CAD build for the part. Positions are in the model's coordinates, mm. Face numbers are marked on the shaded views. A direction names the side the tool comes from. Coordinates: 2 decimals unless noted, no trailing zeros. Write each loop counter-clockwise with the first axis right and the second up, starting at its lowest first coordinate (ties: lowest second). Pieces come first, ordered by that corner, then holes. Notation, with made-up numbers: (-18.5, 50) - (19.5, 50) arc R19 ccw to (19.5, 87) - close; hole circle Ø7 at (-1, 35). An arc over 180 degrees is marked (long way). One line per question, with ' | ' between items. Start each with the question number.
1. Probe line 1 (Y direction, x = -16, z = 24); line 2 (X direction, y = 45, z = 7); line 3 (Y direction, x = -2, z = 27). List the from-to ranges inside material, lowest first.
2. Two-plate mould, pull along Y, no slides. Class the marked faces 1, 2, 3 and 4: +Y half, -Y half, draft (parallel to the pull), parting line (faces both ways), or undercut.
3. Band-saw the part on B-B, the plane x = 13. Write the cut outline in (y, z).
4. Which spindle directions (+Z, -Z, +X, -X, +Y, -Y) get a long thin tool onto all of the face, cutting with end or side? Do the marked faces 5, 6, 7 and 8. Say none if no direction does.
5. Flat gauge pins, fed straight in: P1, Ø2.5, axis at x = -28, y = 35.5, coming from the +Z side; P2, Ø2.5, axis at x = -28, z = 19.5, coming from the -Y side; P3, Ø2.5, axis at x = -27.5, z = 16.5, coming from the +Y side. Where does each tip first touch, or does it go through?
6. Band-saw the part on C-C, the plane x = -19.5. Write the cut outline in (y, z), then the cut area to 3 significant figures.
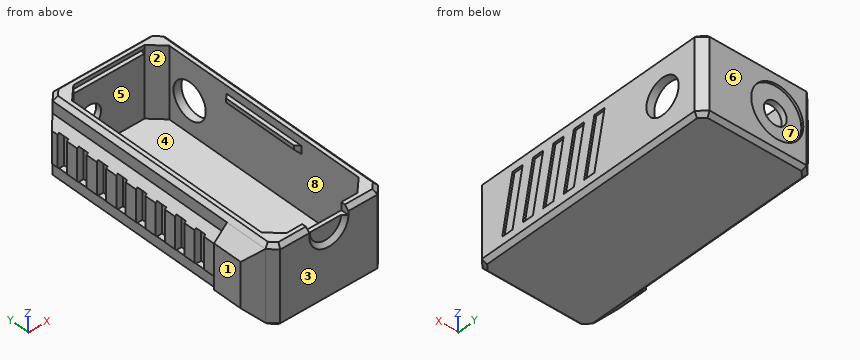
from build123d import *

# Parameters (mm, degrees)
F2_W      = 52
F2_H      = 116
F2_W_2    = 44.8
F2_H_2    = 108.8
F3_DEPTH  = 36
F4_DEPTH  = 3.6
F7_SIZE   = 3.6
F8_SIZE   = 5.9976
F6_R      = 5.25
F9_DEPTH  = 3.6
F5_R      = 8.25
F10_DEPTH = 3.6
F11_W     = 18
F11_H     = 3.6
F12_DEPTH = 3.6
F13_W     = 32.8048
F13_H     = 2
F14_DEPTH = 2.1
F6_R_2    = 12
F15_DEPTH = 1
F16_R     = 0.5
F17_W     = 38.28
F17_H     = 3.6
F19_DEPTH = 1.8
F18_W     = 38.28
F18_H     = 3.6
F20_DEPTH = 1.8
F21_SIZE  = 1.79999
F23_DEPTH = 1.8
F24_SIZE  = 1.79999
F26_W     = 89.2
F26_H     = 21.6
F27_DEPTH = 3.6
F28_DEPTH = 5.9976
F30_SIZE  = 3.59999
F29_W     = 4.775
F29_H     = 15.6718
F31_DEPTH = 2.9972
F32_SIZE  = 5.99759
F34_DEPTH = 0.9


# Not quite as in the source:
# - two fillets or chamfers of one size are made in one step
# - a fillet or chamfer is up to 0.001 mm smaller than in the source, because OpenCascade refuses the exact size


with BuildPart() as f3:
    # F2 (on Top) → F3 (new body)
    with BuildSketch(Plane.XY):
        Rectangle(F2_W, F2_H)
        Rectangle(F2_W_2, F2_H_2, mode=Mode.SUBTRACT)
    extrude(amount=F3_DEPTH)

    # F2 (on Top) → F4 (join)
    with BuildSketch(Plane.XY):
        Rectangle(F2_W_2, F2_H_2)
    extrude(amount=F4_DEPTH)

    # F7
    f7_edges = [f3.edges().sort_by_distance(p)[0] for p in [
        (-26, -58, 18),
        (26, -58, 18),
        (26, 58, 18),
        (-26, 58, 18),
    ]]
    chamfer(f7_edges, length=F7_SIZE)

    # F8
    f8_edges = [f3.edges().sort_by_distance(p)[0] for p in [
        (-22.4, 54.4, 19.8),
        (22.4, 54.4, 19.8),
        (-22.4, -54.4, 19.8),
        (22.4, -54.4, 19.8),
    ]]
    chamfer(f8_edges, length=F8_SIZE)

    # F6 (on face) → F9 (cut)
    with BuildSketch(Plane(origin=(0, 58, 0), x_dir=(-1, 0, 0), z_dir=(0, 1, 0))):
        with Locations((8.84, 18)):
            Circle(F6_R)
    extrude(amount=-F9_DEPTH, mode=Mode.SUBTRACT)

    # F5 (on face) → F10 (cut)
    with BuildSketch(Plane.YZ.offset(26)):
        with Locations((38, 18)):
            Circle(F5_R)
    extrude(amount=-F10_DEPTH, mode=Mode.SUBTRACT)

    # F11 (on face) → F12 (cut)
    with BuildSketch(Plane.XZ.offset(58)):
        with Locations((0, 34.2)):
            Rectangle(F11_W, F11_H)
    extrude(amount=-F12_DEPTH, mode=Mode.SUBTRACT)

    # F13 (on face) → F14 (cut)
    with BuildSketch(Plane.XZ.offset(-54.4)):
        with Locations((0, 33.2)):
            Rectangle(F13_W, F13_H)
    extrude(amount=-F14_DEPTH, mode=Mode.SUBTRACT)

    # F6 (on face) → F15 (cut)
    with BuildSketch(Plane(origin=(0, 58, 0), x_dir=(-1, 0, 0), z_dir=(0, 1, 0))):
        with Locations((8.84, 18)):
            Circle(F6_R_2)
        with Locations((8.84, 18)):
            Circle(F6_R, mode=Mode.SUBTRACT)
    extrude(amount=-F15_DEPTH, mode=Mode.SUBTRACT)

    # F16
    f16_edges = [f3.edges().sort_by_distance(p)[0] for p in [
        (0, 56.5, 34.2),
    ]]
    fillet(f16_edges, radius=F16_R)

    # F17 (on face) → F19 (join)
    with BuildSketch(Plane(origin=(22.4, 0, 0), x_dir=(0, -1, 0), z_dir=(-1, 0, 0))):
        with Locations((0, 30.6)):
            Rectangle(F17_W, F17_H)
    extrude(amount=F19_DEPTH)

    # F18 (on face) → F20 (join)
    with BuildSketch(Plane.YZ.offset(-22.4)):
        with Locations((0, 30.6)):
            Rectangle(F18_W, F18_H)
    extrude(amount=F20_DEPTH)

    # F21 (size 1.8 in the source; OpenCascade refuses exactly that, so slightly less here)
    f21_edges = [f3.edges().sort_by_distance(p)[0] for p in [
        (-20.6, -19.14, 30.6),
        (-20.6, 0, 28.8),
        (-20.6, 19.14, 30.6),
        (20.6, 19.14, 30.6),
        (20.6, 0, 28.8),
        (20.6, -19.14, 30.6),
        (-15.7, -58, 36),
        (-24.2, -56.2, 36),
        (-26, 0, 36),
        (-24.2, 56.2, 36),
        (0, 58, 36),
        (24.2, 56.2, 36),
        (26, 0, 36),
        (24.2, -56.2, 36),
        (15.7, -58, 36),
        (0, -58, 0),
        (-24.2, -56.2, 0),
        (-26, 0, 0),
        (-24.2, 56.2, 0),
        (0, 58, 0),
        (24.2, 56.2, 0),
        (26, 0, 0),
        (24.2, -56.2, 0),
    ]]
    chamfer(f21_edges, length=F21_SIZE)

    # F11 (on face) → F23 (cut)
    with BuildSketch(Plane.XZ.offset(58)):
        with BuildLine():
            ThreePointArc((-9, 32.4), (0, 23.4), (9, 32.4))
            Line((9, 32.4), (-9, 32.4))
        make_face()
    extrude(amount=-F23_DEPTH, mode=Mode.SUBTRACT)

    # F24 (size 1.8 in the source; OpenCascade refuses exactly that, so slightly less here)
    f24_edges = [f3.edges().sort_by_distance(p)[0] for p in [
        (0, -56.2, 23.4),
    ]]
    chamfer(f24_edges, length=F24_SIZE)

    # F26 (on face) → F27 (join)
    with BuildSketch(Plane(origin=(-26, 0, 0), x_dir=(0, -1, 0), z_dir=(-1, 0, 0))):
        with Locations((-9.8, 18)):
            Rectangle(F26_W, F26_H)
    extrude(amount=F27_DEPTH)

    # F26 (on face) → F28 (join)
    with BuildSketch(Plane(origin=(-26, 0, 0), x_dir=(0, -1, 0), z_dir=(-1, 0, 0))):
        Polygon((54.4, 1.8), (54.4, 34.2), (34.8, 34.2), (34.8, 28.8), (34.8, 7.2), (34.8, 1.8), align=None)
    extrude(amount=F28_DEPTH)

    # F30 (size 3.6 in the source; OpenCascade refuses exactly that, so slightly less here)
    f30_edges = [f3.edges().sort_by_distance(p)[0] for p in [
        (-29.6, 54.4, 18),
        (-29.6, 9.8, 7.2),
        (-29.6, 9.8, 28.8),
    ]]
    chamfer(f30_edges, length=F30_SIZE)

    # F29 (on face) → F31 (cut)
    with BuildSketch(Plane(origin=(-29.6, 0, 0), x_dir=(0, -1, 0), z_dir=(-1, 0, 0))):
        with Locations((-45.4, 18)):
            Rectangle(F29_W, F29_H)
        with Locations((-35.395, 18)):
            Rectangle(F29_W, F29_H)
        with Locations((-25.39, 18)):
            Rectangle(F29_W, F29_H)
        with Locations((-15.385, 18)):
            Rectangle(F29_W, F29_H)
        with Locations((-5.38, 18)):
            Rectangle(F29_W, F29_H)
        with Locations((4.625, 18)):
            Rectangle(F29_W, F29_H)
        with Locations((14.63, 18)):
            Rectangle(F29_W, F29_H)
        with Locations((24.635, 18)):
            Rectangle(F29_W, F29_H)
    extrude(amount=-F31_DEPTH, mode=Mode.SUBTRACT)

    # F32 (size 5.9976 in the source; OpenCascade refuses exactly that, so slightly less here)
    f32_edges = [f3.edges().sort_by_distance(p)[0] for p in [
        (-31.9976, -44.6, 34.2),
        (-31.9976, -54.4, 18),
        (-31.9976, -44.6, 1.8),
    ]]
    chamfer(f32_edges, length=F32_SIZE)

    # F33 (on face) → F34 (cut)
    with BuildSketch(Plane.YZ.offset(26)):
        Polygon((-33.4704, 30.7), (-38.7028, 30.7), (-43.9352, 5.3), (-38.7028, 5.3), align=None)
        Polygon((-23.0056, 30.7), (-28.238, 30.7), (-33.4704, 5.3), (-28.238, 5.3), align=None)
        Polygon((-12.5408, 30.7), (-17.7732, 30.7), (-23.0056, 5.3), (-17.7732, 5.3), align=None)
        Polygon((-2.076, 30.7), (-7.3084, 30.7), (-12.5408, 5.3), (-7.3084, 5.3), align=None)
        Polygon((8.3888, 30.7), (3.1564, 30.7), (-2.076, 5.3), (3.1564, 5.3), align=None)
    extrude(amount=-F34_DEPTH, mode=Mode.SUBTRACT)


solid = f3.part
Filled in:
1) line 1: y = -58 to -54.4, 54.4 to 57 | line 2: x = -26 to -22.4, 22.4 to 26 | line 3: y = -56.2 to -54.4, 54.4 to 57
2) face 1: draft | face 2: undercut | face 3: -Y half | face 4: undercut
3) outline: (-58, 1.8) - (-56.2, 0) - (56.2, 0) - (58, 1.8) - (58, 34.2) - (56.2, 36) - (54.4, 36) - (54.4, 34.2) - (56, 34.2) arc R0.5 cw to (56.5, 33.7) - (56.5, 32.2) - (54.4, 32.2) - (54.4, 3.6) - (-54.4, 3.6) - (-54.4, 36) - (-56.2, 36) - (-58, 34.2) - close
4) face 5: +Z | face 6: +Z, -Z, +X, -X, +Y | face 7: +Y | face 8: none
5) P1: stops at z = 28.05 | P2: stops at y = -53.65 | P3: stops at y = 54.15
6) outline: (-58, 1.8) - (-56.2, 0) - (56.2, 0) - (58, 1.8) - (58, 12.49) - (57, 12.49) - (57, 23.51) - (58, 23.51) - (58, 34.2) - (56.2, 36) - (51.3, 36) - (51.3, 3.6) - (-51.3, 3.6) - (-51.3, 36) - (-56.2, 36) - (-58, 34.2) - close | area: 834 mm²
